```python
from build123d import *

# Parameters (mm, degrees)
SKETCH8_R           = 83.841254666
SKETCH8_R_2         = 82.317249201
BOSS_EXTRUDE1_DEPTH = 10.16
SKETCH9_R           = 78.358924529
CUT_EXTRUDE1_DEPTH  = 187.96


with BuildPart() as part:
    # Sketch7 → Revolve3 (revolve)
    with BuildSketch(Plane.XY):
        with BuildLine():
            add(Edge.make_bspline(
                [(2.890004562, 0), (2.895382745, 0.002478586), (3.114731574, 0.103470328), (3.772189671, 0.394557939), (4.892593468, 0.849688542), (6.72155052, 1.53547194), (9.051268741, 2.333090251), (12.826018708, 3.522776414), (17.599278058, 4.890957749), (23.373563661, 6.413247874), (29.176516141, 7.846136382), (36.94300293, 9.663971784), (46.689062936, 11.798346486), (58.424874502, 14.197738172), (70.188922239, 16.473591194), (81.974602451, 18.6463018), (97.71264621, 21.42647714), (117.420654598, 24.716507147), (141.110859364, 28.429826036), (164.833348495, 31.946353837), (188.581698126, 35.293998221), (212.351621104, 38.492682711), (244.069560818, 42.577741353), (283.757517922, 47.375416088), (331.434490554, 52.701690304), (379.154862581, 57.632899759), (426.912731664, 62.191265335), (490.634576058, 67.782687664), (554.417145386, 72.64929345), (618.252364776, 76.709424177), (658.17025028, 78.866656722), (690.115671587, 80.31586406), (714.080440133, 81.240229409), (734.052133379, 81.850150654), (750.032605884, 82.191005794), (758.010055581, 82.306548561), (762, 82.317249201)],
                knots=[0.003470978, 0.003470978, 0.003470978, 0.003470978, 0.00349552, 0.004471529, 0.006423545, 0.008375562, 0.012279595, 0.016183628, 0.023991695, 0.031799761, 0.039607828, 0.047415894, 0.063032027, 0.07864816, 0.094264293, 0.109880426, 0.125496558, 0.156728824, 0.18796109, 0.219193356, 0.250425621, 0.281657887, 0.312890153, 0.375354685, 0.437819216, 0.500283748, 0.562748279, 0.625212811, 0.750141874, 0.812606405, 0.875070937, 0.906303203, 0.937535468, 0.968767734, 0.984383867, 0.999994686, 0.999994686, 0.999994686, 0.999994686], degree=3))
            Line((762, 82.317249201), (762, 83.841254666))
            add(Edge.make_bspline(
                [(0, 0), (0.002469036, 0.007698152), (0.00852038, 0.022545642), (0.025428785, 0.049911406), (0.065694849, 0.100096678), (0.127523873, 0.163176144), (0.212062429, 0.237272493), (0.332279694, 0.331578396), (0.47681638, 0.434147846), (0.646496772, 0.544815952), (0.841412681, 0.663024364), (1.126864222, 0.82633392), (1.572744504, 1.062892156), (2.33539055, 1.432268664), (3.710931738, 2.02979685), (6.154578127, 2.969838304), (10.668005752, 4.490267325), (18.999517068, 6.917303838), (33.385795617, 10.520869917), (58.214680344, 15.881727226), (92.501407111, 22.236378549), (134.347160824, 29.066892837), (181.232321928, 35.913847395), (228.199436648, 42.167572329), (275.229416109, 47.928683924), (322.309575865, 53.261898342), (369.432294544, 58.204857708), (416.591925172, 62.781349507), (463.784734462, 67.002125548), (511.007900045, 70.868414522), (558.259527802, 74.370378395), (605.538293137, 77.485800464), (646.930327879, 79.837294836), (682.425589554, 81.539197971), (710.863439026, 82.65535626), (729.852911101, 83.259007577), (745.309411706, 83.632760833), (754.846503834, 83.785926018), (759.61543609, 83.834878653), (762, 83.841254666)],
                knots=[0, 0, 0, 0, 0, 4.177e-05, 8.3539e-05, 0.000167079, 0.000334158, 0.000501236, 0.000668315, 0.000962463, 0.001256611, 0.001555846, 0.001855081, 0.002674694, 0.003884179, 0.005967022, 0.009661666, 0.016303633, 0.028675652, 0.051140007, 0.0868676, 0.148543873, 0.210220157, 0.271896443, 0.333572727, 0.395249011, 0.456925295, 0.518601581, 0.580277867, 0.641954151, 0.703630435, 0.765306721, 0.826983006, 0.888659291, 0.919497433, 0.950335576, 0.975167788, 0.987583894, 1, 1, 1, 1, 1], degree=4))
            Line((0, 0), (2.890004562, 0))
        make_face()
    revolve(axis=Axis((0, 0, 0), (1, 0, 0)))

    # Sketch8 → Boss-Extrude1 (add)
    with BuildSketch(Plane(origin=(762, 0, 0), x_dir=(0, 0, -1), z_dir=(1, 0, 0))):
        with Locations(Location((0, 0, 0), (0, 0, 90))):
            Circle(SKETCH8_R)
        with Locations(Location((0, 0, 0), (0, 0, 270))):
            Circle(SKETCH8_R_2, mode=Mode.SUBTRACT)
    extrude(amount=BOSS_EXTRUDE1_DEPTH)

    # Sketch9 → Cut-Extrude1 (cut)
    with BuildSketch(Plane(origin=(162.56, 0, 0), x_dir=(0, 0, -1), z_dir=(1, 0, 0))):
        Circle(SKETCH9_R)
    extrude(amount=-CUT_EXTRUDE1_DEPTH, mode=Mode.SUBTRACT)


solid = part.part
```
Model file for the job. Use its own axes, mm. Coordinates: 2 decimals unless noted, no trailing zeros. Return JSON: item names as keys, results as strings. Group by question number.
1) Probe line 1 (Z direction, x = 766, y = 0); line 2 (Z direction, x = 686.5, y = -47); line 3 (Y direction, x = 712, z = -39). List the from-to ranges inside material, lowest first. Write a range as from..to.
2) Mould opens along Z. For faces 1 (the flat face through (162.56, -27, -17)), 2 (the cylindrical face through (767.01, 77.45, -32.11)), 3 (the cylindrical face through (767.009, 82.238, -3.619)) say: released by +Z, released by -Z, zero draft, split by the parting line, or undercut.
3) Flat gauge pins, fed straight in: P1, Ø10, axis at x = 392.5, y = 44.5, coming from the +Z side; P2, Ø2, axis at x = 480.5, z = 35.5, coming from the -Y side; P3, Ø12, axis at x = 382.5, y = 42, coming from the +Z side. Where does each tip first touch, or does it go through?
Values found:
{
 "1": {"line 1": "z = -83.84..-82.32, 82.32..83.84", "line 2": "z = -66.78..-64.9, 64.9..66.78", "line 3": "y = -72.88..-71.15, 71.15..72.88"},
 "2": {"face 1": "zero draft", "face 2": "split by the parting line", "face 3": "undercut"},
 "3": {"P1": "stops at z = 45.76", "P2": "stops at y = -59", "P3": "stops at z = 47.35"}
}
